CAD build for the part. Positions are in the model's coordinates, mm. Coordinates: 2 decimals unless noted, no trailing zeros. Write each loop counter-clockwise with the first axis right and the second up, starting at its lowest first coordinate (ties: lowest second). Pieces come first, ordered by that corner, then holes.
Autodesk Inventor part; units mm, degrees
ref_plane "YZ Plane" through (0, 0, 0) normal (1, 0, 0) x (0, 1, 0)
ref_plane "XZ Plane" through (0, 0, 0) normal (0, 1, 0) x (-1, 0, 0)
ref_plane "XY Plane" through (0, 0, 0) normal (0, 0, 1) x (1, 0, 0)
sketch "Sketch1" plane through (0, 0, 0) normal (0, 0, 1) x (1, 0, 0)
  line L0 (-86, 40) -> (-86, 90)
  line L1 (-86, 90) -> (304, 90)
  line L2 (304, 90) -> (304, 40)
  circle A0 centre (72, 63) radius 8
  circle A1 centre (147, 78) radius 4
  circle A2 centre (-3, 78) radius 4
  line L3 (-86, 40) -> (304, 40)
  circle A3 centre (-58, 65) radius 3
  circle A4 centre (276, 65) radius 3
  circle A5 centre (109, 65) radius 3
  dimension "d1" = 390
  dimension "d2" = 16
  dimension "d6" = 8
  dimension "d7" = 8
  dimension "d8" = 15
  dimension "d13" = 75
  dimension "d14" = 75
  dimension "d27" = 15
  dimension "d38" = 50
  dimension "d58" = 27
  dimension "d68" = 232
  dimension "d69" = 6
  dimension "d70" = 25
  dimension "d71" = 28
  dimension "d72" = 6
  dimension "d73" = 25
  dimension "d74" = 28
  dimension "d75" = 6
  dimension "d76" = 25
  dimension "d77" = 195
extrude "Extrusión3" add sketch "Sketch1" along normal blind 10
sketch "Boceto3" plane through (304, 40, 0) normal (1, 0, 0) x (0, 0, -1)
  line L0 (-10, 0) -> (-10, 50)
  line L1 (-10, 50) -> (-5, 50)
  line L2 (0, 50) -> (-10, 50)
  line L3 (0, 0) -> (0, 50)
  line L4 (-5, 0) -> (-5, 12.5)
  line L5 (-5, 50) -> (-5, 37.5)
  circle A0 centre (-5, 37.5) radius 3
  circle A1 centre (-5, 12.5) radius 3
  point P0 (0, -40)
  dimension "d42" = 5
  dimension "d43" = 50
  dimension "d44" = 12.5
  dimension "d45" = 12.5
  dimension "d46" = 6
  dimension "d47" = 6
extrude "Extrusión4" cut sketch "Boceto3" against normal blind 15
sketch "Boceto4" plane through (-86, 40, 0) normal (-1, 0, 0) x (0, 0, 1)
  line L0 (10, 0) -> (10, 50)
  line L1 (10, 50) -> (5, 50)
  line L2 (0, 50) -> (10, 50)
  line L3 (5, 50) -> (5, 0)
  line L4 (5, 0) -> (5, 12.5)
  line L5 (5, 50) -> (5, 37.5)
  circle A0 centre (5, 12.5) radius 3
  circle A1 centre (5, 37.5) radius 3
  point P0 (0, -40)
  dimension "d50" = 5
  dimension "d51" = 50
  dimension "d52" = 12.5
  dimension "d53" = 12.5
extrude "Extrusión5" cut sketch "Boceto4" against normal blind 15
thread "Rosca1"
thread "Rosca2"
thread "Rosca3"
thread "Rosca4"
thread "Rosca5"
thread "Rosca6"
thread "Rosca7"
equation "\"d73\" = d70"
equation "\"d74\" = d71"
equation "\"d76\" = d70"
properties part number "Frente" material "Aluminio 6061"
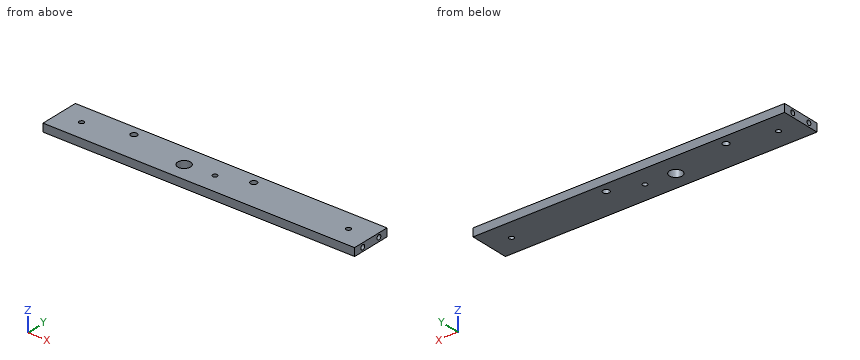
Item 1: Wall check: line 1 along Y through (x, z) = (300.75, 5); line 2 along Y through (x, z) = (276, 4.5); line 3 along X through (y, z) = (75.5, 9.75). Give the ranges that are in metal, low to high.
Item 2: Saw through at A-A, the plane z = 5. Write the cut outline in (x, y).
Item 3: Saw through at C-C, the plane x = -3. Write the cut outline in (y, z), and give its area (3 significant figures).
Item 4: Saw through at B-B, the plane x = 72. Write the cut outline in (y, z), and give its area (3 significant figures).
Item 5: Flat gauge pin, fed straight in: pin 1 Ø5 at (y, z) = (52.5, 5) entering from +X. Where does the tip first touch, or does it go through?
Working result:
1. line 1: y = 40 to 49.5, 55.5 to 74.5, 80.5 to 90
1. line 2: y = 40 to 62, 68 to 90
1. line 3: x = -86 to -6.12, 0.12 to 143.88, 150.12 to 304
2. outline: (-86, 40) - (304, 40) - (304, 49.5) - (289, 49.5) - (289, 55.5) - (304, 55.5) - (304, 74.5) - (289, 74.5) - (289, 80.5) - (304, 80.5) - (304, 90) - (-86, 90) - (-86, 80.5) - (-71, 80.5) - (-71, 74.5) - (-86, 74.5) - (-86, 55.5) - (-71, 55.5) - (-71, 49.5) - (-86, 49.5) - close; hole circle Ø6 at (-58, 65); hole circle Ø8 at (-3, 78); hole circle Ø16 at (72, 63); hole circle Ø6 at (109, 65); hole circle Ø8 at (147, 78); hole circle Ø6 at (276, 65)
3. outline: (40, 0) - (74, 0) - (74, 10) - (40, 10) - close; (82, 0) - (90, 0) - (90, 10) - (82, 10) - close
3. area: 420 mm2
4. outline: (40, 0) - (55, 0) - (55, 10) - (40, 10) - close; (71, 0) - (90, 0) - (90, 10) - (71, 10) - close
4. area: 340 mm2
5. pin 1: stops at x = 289
